```python
from build123d import *

# Parameters (mm, degrees)
EXTRUDE_1_DEPTH     = 15
SKETCH_9_R          = 10
CUT_EXTRUDE_3_DEPTH = 2


with BuildPart() as part:
    # ｽｹｯﾁ4 → ﾎﾞｽ - 押し出し1 (new body)
    with BuildSketch(Plane.XY):
        with BuildLine():
            Line((-53.623111018, -124.995132678), (-58.940636287, -129.45706617))
            ThreePointArc((-58.940636287, -129.45706617), (-60.005384698, -131.552012131), (-59.233530865, -133.771635843))
            ThreePointArc((-59.233530865, -133.771635843), (57.362306223, -135.763481103), (52.076178918, -19.270504783))
            Line((52.076178918, -19.270504783), (10.606601718, 10.606601718))
            ThreePointArc((10.606601718, 10.606601718), (-10.606601718, 10.606601718), (-10.606601718, -10.606601718))
            Line((-10.606601718, -10.606601718), (14.536280154, -62.889638219))
            ThreePointArc((14.536280154, -62.889638219), (14.918089499, -66.109676181), (13.244185189, -68.886809092))
            Line((13.244185189, -68.886809092), (-53.623111018, -124.995132678))
        make_face()
        with BuildLine():
            Line((21.232400696, -76.813798404), (45.844843506, -127.993820346))
            ThreePointArc((45.844843506, -127.993820346), (46.221944165, -131.235480845), (44.518718993, -134.019289696))
            ThreePointArc((44.518718993, -134.019289696), (-2.231208213, -149.964431749), (-47.870174388, -131.072951785))
            ThreePointArc((-47.870174388, -131.072951785), (-48.817477846, -128.802229421), (-47.747678417, -126.586582094))
            Line((-47.747678417, -126.586582094), (13.511229465, -75.151532228))
            ThreePointArc((13.511229465, -75.151532228), (17.77869109, -74.092739753), (21.232400696, -76.813798404))
        make_face(mode=Mode.SUBTRACT)
    extrude(amount=EXTRUDE_1_DEPTH)

    # ｽｹｯﾁ9 → ｶｯﾄ - 押し出し3 (cut)
    with BuildSketch(Plane(origin=(0, 0, 0), x_dir=(-1, 0, 0), z_dir=(0, 0, -1))):
        Circle(SKETCH_9_R)
    extrude(amount=-CUT_EXTRUDE_3_DEPTH, mode=Mode.SUBTRACT)


solid = part.part
```
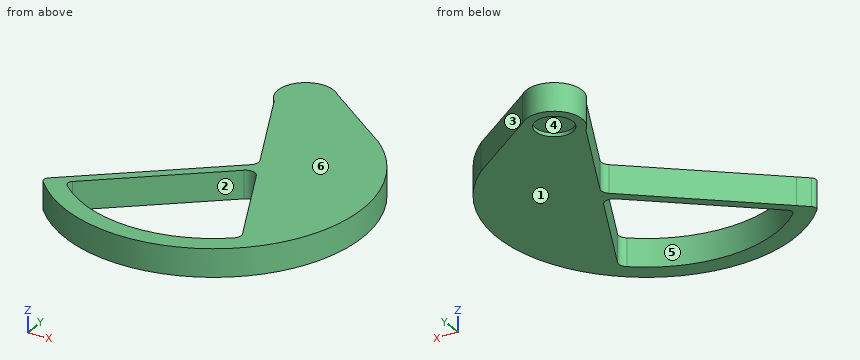
CAD build for the part. Positions are in the model's coordinates, mm. Face numbers are marked on the shaded views. A direction names the side the tool comes from. Coordinates: 2 decimals unless noted, no trailing zeros. Write each loop counter-clockwise with the first axis right and the second up, starting at its lowest first coordinate (ties: lowest second). Pieces come first, ordered by that corner, then holes.
(1) Flat gauge pins, fed straight in: pin 1 (4 mm diameter, centred on y = -122.5, z = 12, fed in from +X); pin 2 (22 mm diameter, centred on x = 3, y = 2, fed in from -Z); pin 3 (1 mm diameter, centred on y = -78.5, z = 6.5, fed in from +X); pin 4 (6 mm diameter, centred on y = -75, z = 6, fed in from -X). Where does each tip first touch, or does it go through?
(2) Cut at A-A, the plane x = -32.5. List the corners of the cut face in (y, z), and give its area (3 significant figures).
(3) Cut at C-C, the plane x = 2.5. List the corners of the cut face in (y, z), and give its area (3 significant figures).
(4) Drill centre lines: probe 1 along Y at (x, z) = (0, 0.8); probe 2 along Y at (x, z) = (3, 1); probe 3 along Y at (x, z) = (-41.5, 13). Where is each one in solid material? Low to high.
(5) Cut at B-B, the plane z = 7.5. List the corners of the cut face in (x, y).
(6) Cut at D-D, the plane y = -80. List the corners of the cut face in (x, z), and give its area (3 significant figures).
(7) Two-plate mould, pull along Y, no slides. Class the marked faces 1, 2 and 3: +Y half, -Y half, draft (parallel to the pull), parting line (faces both ways), or undercut.
(8) 3-axis set-ups, long thin cutter, end or side, ignore diameter. For the marked faces 4, 5 and 6: which of +Z, -Z, +X, -X, +Y, -Y reach the whole face in a straight line?
Geometry says:
1. pin 1: stops at x = 68.99
1. pin 2: stops at z = 0
1. pin 3: stops at x = 79.99
1. pin 4: stops at x = 2.38
2. outline: (-153.1, 0) - (-142, 0) - (-142, 15) - (-153.1, 15) - close; (-113.78, 0) - (-107.27, 0) - (-107.27, 15) - (-113.78, 15) - close
2. area: 264 mm2
3. outline: (-159.96, 0) - (-149.96, 0) - (-149.96, 15) - (-159.96, 15) - close; (-84.4, 0) - (-77.9, 0) - (-77.9, 15) - (-84.4, 15) - close; (-37.86, 0) - (-9.68, 0) - (-9.68, 2) - (9.68, 2) - (9.68, 0) - (14.79, 0) - (14.79, 15) - (-37.86, 15) - close
3. area: 999 mm2
4. probe 1: y = -160 to -150, -86.5 to -80, -32.66 to -10, 10 to 15
4. probe 2: y = -159.94 to -149.94, -83.98 to -77.48, -38.9 to -9.54, 9.54 to 14.7
4. probe 3: y = -148.39 to -136.37, -121.34 to -114.82
5. outline: (-59.23, -133.77) arc R80 ccw (long way) to (52.08, -19.27) - (10.61, 10.61) arc R15 ccw to (-10.61, -10.61) - (14.54, -62.89) arc R5 cw to (13.24, -68.89) - (-58.94, -129.46) arc R3 ccw to start; hole (-47.87, -131.07) arc R70 ccw to (44.52, -134.02) arc R5 ccw to (45.84, -127.99) - (21.23, -76.81) arc R5 ccw to (13.51, -75.15) - (-47.75, -126.59) arc R3 ccw to start
6. outline: (0, 0) - (7.74, 0) - (7.74, 15) - (0, 15) - close; (22.76, 0) - (80, 0) - (80, 15) - (22.76, 15) - close
6. area: 975 mm2
7. face 1: draft
7. face 2: undercut
7. face 3: +Y half
8. face 4: -Z
8. face 5: +Z, -Z
8. face 6: +Z, +X, -X, +Y, -Y
